Geometry: final body of the model. Coordinates: model frame, mm. Coordinates: 2 decimals unless noted, no trailing zeros. Order: outer loops, then holes, each group sorted by start corner. A loop starts at its lowest first (then second) coordinate and runs counter-clockwise, first axis right, second up. Notation, with made-up numbers: M -4,33.5 L 52,33.5 A23 ccw 52,60.5 Z; hole C -5,66.25 d6. An arc over 180 degrees is marked long. One line per question, with ' | ' between items.
from build123d import *

# Parameters (mm, degrees)
SKETCH1_R           = 2.3
BOSS_EXTRUDE1_DEPTH = 3


with BuildPart() as part:
    # Sketch1 → Boss-Extrude1 (new body)
    with BuildSketch(Plane(origin=(0, 0, 0), x_dir=(1, 0, 0), z_dir=(0, 1, 0))):
        with BuildLine():
            Line((3.409188309, -5.24766594), (5.24766594, -3.409188309))
            ThreePointArc((5.24766594, -3.409188309), (5.781490388, -2.39477173), (6.121320344, -1.3))
            Line((6.121320344, -1.3), (6.121320344, 1.3))
            ThreePointArc((6.121320344, 1.3), (5.781490388, 2.39477173), (5.24766594, 3.409188309))
            Line((5.24766594, 3.409188309), (3.409188309, 5.24766594))
            ThreePointArc((3.409188309, 5.24766594), (2.39477173, 5.781490388), (1.3, 6.121320344))
            Line((1.3, 6.121320344), (-1.3, 6.121320344))
            ThreePointArc((-1.3, 6.121320344), (-2.39477173, 5.781490388), (-3.409188309, 5.24766594))
            Line((-3.409188309, 5.24766594), (-5.24766594, 3.409188309))
            ThreePointArc((-5.24766594, 3.409188309), (-5.781490388, 2.39477173), (-6.121320344, 1.3))
            Line((-6.121320344, 1.3), (-6.121320344, -1.3))
            ThreePointArc((-6.121320344, -1.3), (-5.781490388, -2.39477173), (-5.24766594, -3.409188309))
            Line((-5.24766594, -3.409188309), (-3.409188309, -5.24766594))
            ThreePointArc((-3.409188309, -5.24766594), (-2.39477173, -5.781490388), (-1.3, -6.121320344))
            Line((-1.3, -6.121320344), (1.3, -6.121320344))
            ThreePointArc((1.3, -6.121320344), (2.39477173, -5.781490388), (3.409188309, -5.24766594))
        make_face()
        with Locations(Location((0, 0, 0), (0, 0, 270))):
            Circle(SKETCH1_R, mode=Mode.SUBTRACT)
    extrude(amount=-BOSS_EXTRUDE1_DEPTH)


solid = part.part
1. Draft query along X for faces 1 (the face through (0.691, -1.479, 2.194)), 2 (the face through (-2.38, -1.479, -5.788)), 3 (the face through (0, 0, -3)). Return one class per face: pulls with the +X half, pulls with the -X half, needs draft (parallel to the pull), parting line crosses it, or undercut.
Response values:
face 1: undercut | face 2: pulls with the -X half | face 3: needs draft
2. Section D-D, the plane z = 5. Output: boundary loops of the cut face in (x, y), and give its area (3 significant figures).
Response values:
outline: M -3.66,-3 L 3.66,-3 L 3.66,0 L -3.66,0 Z | area: 21.9 mm^2
3. Section C-C, the plane x = 0. Output: boundary loops of the cut face in (y, z), and give its area (3 significant figures).
Response values:
outline: M -3,-6.12 L 0,-6.12 L 0,-2.3 L -3,-2.3 Z; M -3,2.3 L 0,2.3 L 0,6.12 L -3,6.12 Z | area: 22.9 mm^2
4. Section B-B, the plane y = -1.8. Output: boundary loops of the cut face in (x, z).
Response values:
outline: M -6.12,-1.3 A6.26 ccw -5.25,-3.41 L -3.41,-5.25 A6.26 ccw -1.3,-6.12 L 1.3,-6.12 A6.26 ccw 3.41,-5.25 L 5.25,-3.41 A6.26 ccw 6.12,-1.3 L 6.12,1.3 A6.26 ccw 5.25,3.41 L 3.41,5.25 A6.26 ccw 1.3,6.12 L -1.3,6.12 A6.26 ccw -3.41,5.25 L -5.25,3.41 A6.26 ccw -6.12,1.3 Z; hole C 0,0 d4.6
5. Section A-A, the plane z = 0. Output: boundary loops of the cut face in (x, y), and give its area (3 significant figures).
Response values:
outline: M -6.12,-3 L -2.3,-3 L -2.3,0 L -6.12,0 Z; M 2.3,-3 L 6.12,-3 L 6.12,0 L 2.3,0 Z | area: 22.9 mm^2
6. Material intervals for line 1 (X direction, y = -1.9, z = 0); line 2 (X direction, y = -0.2, z = 0.75); line 3 (Z direction, x = 4.5, y = -0.3), sorted ascending. Write a range as [from, to].
Response values:
line 1: x = [-6.12, -2.3], [2.3, 6.12] | line 2: x = [-6.12, -2.17], [2.17, 6.12] | line 3: z = [-4.16, 4.16]
7. Pin query (flat end, axial travel): P1, Ø1, axis at x = -4, y = -2, coming from the -Z side; P2, Ø6, axis at x = 0, z = 0, coming from the +Y side. Return the tip coordinate at first contact, or that it passes through.
Response values:
P1: stops at z = -5.16 | P2: stops at y = 0
